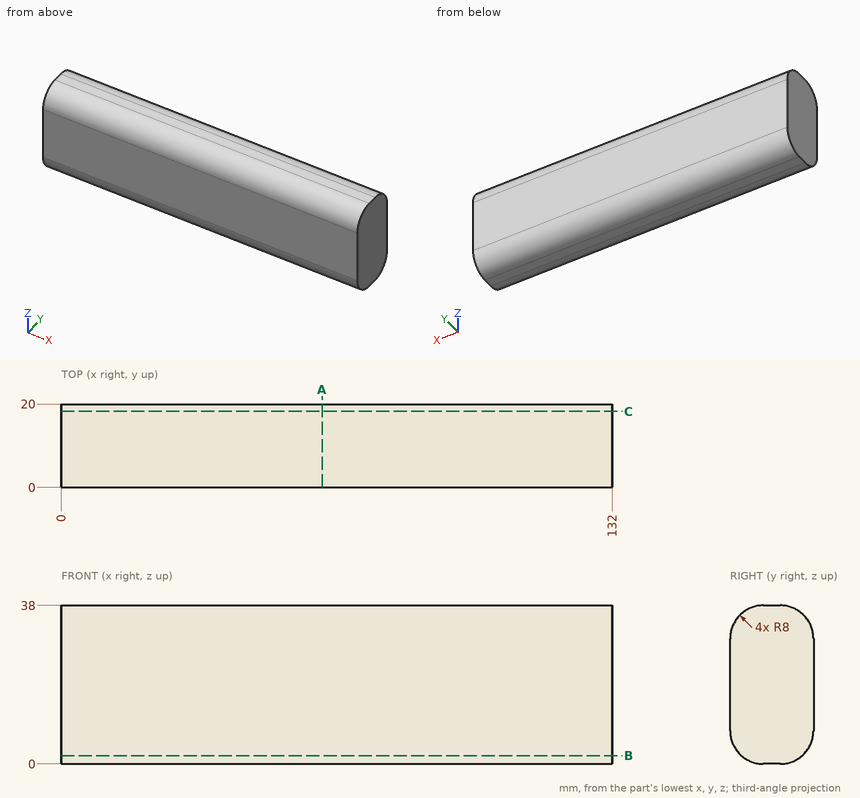
Geometry: see drawing. Coordinates: mm, zero at the bounding-box minimum. Coordinates: 2 decimals unless noted, no trailing zeros. Loops run counter-clockwise (first coordinate to the right, second up) from the corner with the lowest first, then second, coordinate; pieces in that order, holes last.
(1) Material intervals for probe 1 along Z at (x, y) = (117, 3.5); probe 2 along Z at (x, y) = (120.5, 18.75); probe 3 along Y at (x, z) = (67, 32), sorted ascending.
(2) Section B-B on z = 2. Return the cut outline in (x, y), then the cut area to 3 significant figures.
(3) First-contact query: pin 1 Ø2 at (x, y) = (54.5, 17.5) entering from -Z; pin 2 Ø1 at (x, y) = (85, 13.5) entering from -Z; pin 3 Ø1.5 at (x, z) = (77.5, 32) entering from +Y. Flat tips, straight axial feed; report the tip coordinate or a pass-through.
(4) Section A-A on x = 62.5. Return the cut outline in (y, z), then the cut area to 3 significant figures.
(5) Section C-C on y = 18.25. Return the cut outline in (x, z), then the cut area to 3 significant figures.
Data:
1. probe 1: z = 1.39 to 36.61
1. probe 2: z = 3.71 to 34.29
1. probe 3: y = 0.25 to 19.75
2. outline: (0, 2.71) - (132, 2.71) - (132, 17.29) - (0, 17.29) - close
2. area: 1,920 mm2
3. pin 1: stops at z = 1.39
3. pin 2: stops at z = 0.06
3. pin 3: stops at y = 19.9
4. outline: (0, 8) arc R8 ccw to (8, 0) - (12, 0) arc R8 ccw to (20, 8) - (20, 30) arc R8 ccw to (12, 38) - (8, 38) arc R8 ccw to (0, 30) - close
4. area: 705 mm2
5. outline: (0, 3.01) - (132, 3.01) - (132, 34.99) - (0, 34.99) - close
5. area: 4,220 mm2
